The model under review builds one solid part; all positions refer to its coordinate system, in mm. Round coordinates to 2 decimals unless told otherwise and drop trailing zeros. Write each loop counter-clockwise with the first axis right and the second up, starting at its lowest first coordinate (ties: lowest second). Pieces come first, ordered by that corner, then holes. Notation, with made-up numbers: M 15,0 L 68,0 A26 ccw 68,15 Z; hole C 83,64 d11. An arc over 180 degrees is marked long. Write item = value, one per line. Start each with the question number.
Item 1: Take a section at A-A, the plane x = 288.5. Give the boundary of the cut face in (y, z).
Item 2: To check wall thickness, follow line 1 along Y through (x, z) = (336.5, -7.5); line 2 along Z through (x, y) = (310.5, -78); line 3 along Z through (x, y) = (274, -72). State the ranges of each line that lie inside material, in increasing order.
Item 3: For pin 1 Ø3 at (x, z) = (340.5, -4) entering from -Y, flat-tipped, find the tip position at first contact; note if it passes through.
from build123d import *

# Parameters (mm, degrees)
RIGHT_PALM_PAD_DEPTH        = 25
RIGHT_PALM_WEDGE_DEPTH      = 5.38135
RIGHT_PALM_WEDGE_DEPTH_BACK = 191.308
RIGHT_PALM_FILLET_R         = 3


with BuildPart() as part:
    # Right_Palm_Base → Right_Palm_Pad (new body)
    with BuildSketch(Plane.XY.offset(-18)):
        with BuildLine():
            Line((-0.38035, -90.791), (186.307, -90.791))
            ThreePointArc((186.307, -90.791), (189.842534, -89.326534), (191.307, -85.791))
            Line((191.307, -85.791), (191.307, -15.791))
            ThreePointArc((191.307, -15.791), (189.842534, -12.255466), (186.307, -10.791))
            Line((186.307, -10.791), (-0.38035, -10.791))
            ThreePointArc((-0.38035, -10.791), (-3.915884, -12.255466), (-5.38035, -15.791))
            Line((-5.38035, -15.791), (-5.38035, -85.791))
            ThreePointArc((-5.38035, -85.791), (-3.915884, -89.326534), (-0.38035, -90.791))
        make_face()
    extrude(amount=RIGHT_PALM_PAD_DEPTH)

    # Right_Palm_WedgeCut → Right_Palm_Wedge (cut, two sides)
    with BuildSketch(Plane.YZ) as right_palm_wedge_sk:
        Polygon((-45.791, 7), (-92.791, -6), (-92.791, 9), (-45.791, 9), align=None)
    extrude(amount=-RIGHT_PALM_WEDGE_DEPTH, mode=Mode.SUBTRACT)
    extrude(right_palm_wedge_sk.sketch, amount=RIGHT_PALM_WEDGE_DEPTH_BACK, mode=Mode.SUBTRACT)

    # Right_Palm_Fillet
    right_palm_fillet_edges = [part.edges().sort_by_distance(p)[0] for p in [
        (92.963325, -90.791, -5.446809),
        (189.874947, -89.293821, -5.032695),
        (92.963325, -45.791, 7),
        (-5.38035, -65.791, 1.468085),
        (-3.948297, -89.293821, -5.032695),
        (191.307, -65.791, 1.468085),
        (191.307, -30.791, 7),
        (189.842534, -12.255466, 7),
        (92.963325, -10.791, 7),
        (-3.915884, -12.255466, 7),
        (-5.38035, -30.791, 7),
    ]]
    fillet(right_palm_fillet_edges, radius=RIGHT_PALM_FILLET_R)


with BuildPart() as part_1:
    # Right_Palm_Rest placement: moved
    add(part.part.moved(Location((174.06235, 0, 0))))


solid = part_1.part
Response values:
q1.outline = M -90.79,-18 L -10.79,-18 L -10.79,4 A3 ccw -13.79,7 L -45.38,7 A3 ccw -46.18,6.89 L -88.59,-4.84 A3 ccw -90.79,-7.73 Z
q2.line_1 = -90.78 to -10.79
q2.line_2 = -18 to -1.91
q2.line_3 = -18 to -0.25
q3.pin_1 = -89.8
